from build123d import *

# Parameters (mm, degrees)
ESTRUSIONE_ESTRUSIONE1_DEPTH = 30
FORO_PER_VITE_M4_1_D         = 4.5
FORO_PER_VITE_M4_1_DEPTH     = 30
FORO_PER_VITE_M4_1_TIP       = 1.351936393


with BuildPart() as part:
    # Schizzo1 → Estrusione-Estrusione1 (new body)
    with BuildSketch(Plane.XY):
        Polygon((11, -27.5), (11, 17.5), (5, 17.5), (5, 0), (-5, 0), (-5, 17.5), (-11, 17.5), (-11, -27.5), (-5, -27.5), (-5, -10), (5, -10), (5, -27.5), align=None)
    extrude(amount=ESTRUSIONE_ESTRUSIONE1_DEPTH)

    # Foro per Vite M4-1
    with Locations(Plane(origin=(-11, -17.5, 22.5), x_dir=(0, -1, 0), z_dir=(-1, 0, 0))):
        with Locations((0, 0), (0, -15)):
            Hole(FORO_PER_VITE_M4_1_D / 2, depth=FORO_PER_VITE_M4_1_DEPTH)
            with Locations((0, 0, -(FORO_PER_VITE_M4_1_DEPTH + FORO_PER_VITE_M4_1_TIP / 2))):  # 118° drill point
                Cone(0, FORO_PER_VITE_M4_1_D / 2, FORO_PER_VITE_M4_1_TIP, mode=Mode.SUBTRACT)


solid = part.part
Could you check a few things on this model? Use its own coordinates, in mm. A direction names the side the tool comes from. Give positions to 0.01 mm unless a question says otherwise; leave off trailing zeros. Write each loop counter-clockwise with the first axis right and the second up, starting at its lowest first coordinate (ties: lowest second). Pieces come first, ordered by that corner, then holes. Notation, with made-up numbers: (7.25, -11.75) -> (31.25, -11.75) arc R22 ccw to (31.25, 21.25) -> close; hole circle Ø1 at (51, 61). An arc over 180 degrees is marked (long way). Answer as CSV lines item,"result". Start each with the question number.
(1) If we section it at A-A, the plane y = 10.5: Write out the boundary of the cut face in (x, z).
(2) Which directions (+Z, -Z, +X, -X, +Y, -Y) give clear straight access to the entire face, cutting with the end or side of a thin tool? Please do faces 1 (the face through (-5, 9, 15)), 2 (the face through (8.042, -15.354, 8.176)), 3 (the face through (5, -19, 15)).
(3) If we section it at D-D, the plane z = 26.25: Write out the boundary of the cut face in (x, y).
(4) If we section it at B-B, the plane z = 22.5: Write out the boundary of the cut face in (x, y).
(5) I'm going to push flat-ended pins straight in: pin 1 Ø8 at (x, z) = (0, 13.5) entering from -Y; pin 2 Ø8 at (x, z) = (-0.5, 21.5) entering from +Y; pin 3 Ø2.5 at (y, z) = (-17.5, 7.5) entering from -X. Where does each tip first touch, or does it pass through?
(6) If we mould it in two halves opening along X, with no side actions, what happens to faces 4 (the face through (0, -5, 30)), 5 (the face through (-11, -5, 15)), 6 (the face through (0, -10, 15))? For each: +X half, -X half, draft (parallel to the pull), parting line (faces both ways), or undercut.
(7) Please list where these lines run through material, in increasing order: line 1 (Z direction, x = -9.25, y = -17.5); line 2 (X direction, y = 15, z = 23); line 3 (Y direction, x = 3.25, z = 11).
(8) If we section it at C-C, the plane x = -6: Write out the boundary of the cut face in (y, z).
Answer list:
1,outline,"(-11, 0) -> (-5, 0) -> (-5, 30) -> (-11, 30) -> close; (5, 0) -> (11, 0) -> (11, 30) -> (5, 30) -> close"
2,face 1,"+Z, -Z, +Y"
2,face 2,"+X, -X"
2,face 3,"+Z, -Z, -Y"
3,outline,"(-11, -27.5) -> (-5, -27.5) -> (-5, -10) -> (5, -10) -> (5, -27.5) -> (11, -27.5) -> (11, 17.5) -> (5, 17.5) -> (5, 0) -> (-5, 0) -> (-5, 17.5) -> (-11, 17.5) -> close"
4,outline,"(-11, -27.5) -> (-5, -27.5) -> (-5, -19.75) -> (-11, -19.75) -> close; (-11, -15.25) -> (-5, -15.25) -> (-5, -10) -> (5, -10) -> (5, -15.25) -> (11, -15.25) -> (11, 17.5) -> (5, 17.5) -> (5, 0) -> (-5, 0) -> (-5, 17.5) -> (-11, 17.5) -> close; (5, -27.5) -> (11, -27.5) -> (11, -19.75) -> (5, -19.75) -> close"
5,pin 1,"y = -10"
5,pin 2,"y = 0"
5,pin 3,"through"
6,face 4,"draft"
6,face 5,"-X half"
6,face 6,"undercut"
7,line 1,"0 to 5.25, 9.75 to 20.25, 24.75 to 30"
7,line 2,"-11 to -5, 5 to 11"
7,line 3,"-10 to 0"
8,outline,"(-27.5, 0) -> (17.5, 0) -> (17.5, 30) -> (-27.5, 30) -> close; hole circle Ø4.5 at (-17.5, 7.5); hole circle Ø4.5 at (-17.5, 22.5)"
